Check sheet for the modelled part. Datum: model origin and axes. Units: mm. Face numbers are marked on the shaded views. A direction names the side the tool comes from. Round coordinates to 2 decimals unless told otherwise and drop trailing zeros. Order: outer loops, then holes, each group sorted by start corner. A loop starts at its lowest first (then second) coordinate and runs counter-clockwise, first axis right, second up. Notation, with made-up numbers: M -10,16.25 L 7,16.25 A24 ccw 7,31.25 Z; hole C 20,82.5 d3. An arc over 180 degrees is marked long. One line per item, written item: value. Start each with the question number.
(1) Release check for a two-part mould opening along Y. For the marked faces 5, 6 and 7 record: released by +Y, released by -Y, zero draft, split by the parting line, or undercut.
(2) Cross-section at B-B, the plane y = 6.5. Count the separate pieces of the cut face and the enclosed holes in it, and give its area (3 significant figures).
(3) Cross-section at A-A, the plane x = -17. Enter the section's corners in (y, z).
(4) Access from +Z, -Z, +X, -X, +Y, -Y to the whole of each face (thin tool, end or side, straight path). Record for the marked faces 1, 2, 3 and 4.
(5) Thickness scan on L1, parallel to Z at x = 2.65, y = 0; L2, parallel to Y at x = -3.4, z = 29.5; L3, parallel to Y at x = 38, z = 1. Record the ranges inside material, lowest first.
(6) Depth check by flat-ended pin: pin 1 Ø8 at (y, z) = (2, 11.5) entering from +X; pin 2 Ø8 at (y, z) = (2, 31.5) entering from -X; pin 3 Ø5 at (y, z) = (-3, 10) entering from -X. Enter the tip coordinate at first touch or a pass-through.
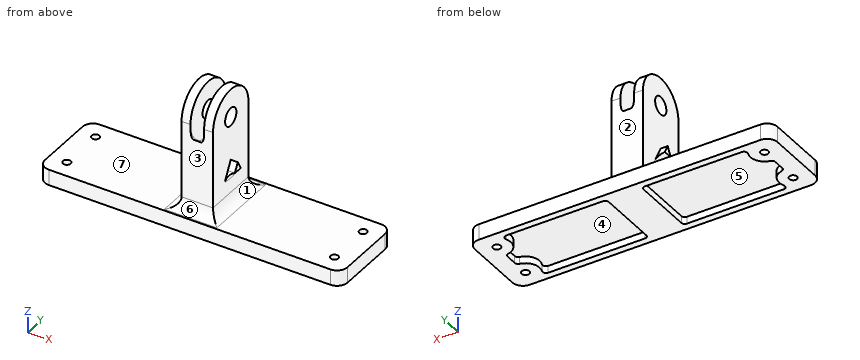
from build123d import *

# Parameters (mm, degrees)
SKETCH1_W           = 86.5
SKETCH1_H           = 23
SKETCH1_R           = 1.1
BOSS_EXTRUDE1_DEPTH = 4.5
CUT_EXTRUDE1_DEPTH  = 2
SKETCH3_R           = 2.55
BOSS_EXTRUDE2_DEPTH = 4.5
SKETCH6_R           = 9
CUT_EXTRUDE3_DEPTH  = 1.95
FILLET1_R           = 3
FILLET2_R           = 1
FILLET3_R           = 1
BOSS_EXTRUDE3_DEPTH = 2
FILLET4_R           = 3


with BuildPart() as part:
    # Sketch1 → Boss-Extrude1 (new body)
    with BuildSketch(Plane.XY):
        Rectangle(SKETCH1_W, SKETCH1_H)
        with Locations((38.25, 6.5)):
            Circle(SKETCH1_R, mode=Mode.SUBTRACT)
        with Locations((38.25, -6.5)):
            Circle(SKETCH1_R, mode=Mode.SUBTRACT)
        with Locations((-38.25, -6.5)):
            Circle(SKETCH1_R, mode=Mode.SUBTRACT)
        with Locations((-38.25, 6.5)):
            Circle(SKETCH1_R, mode=Mode.SUBTRACT)
    extrude(amount=BOSS_EXTRUDE1_DEPTH)

    # Sketch2 → Cut-Extrude1 (cut)
    with BuildSketch(Plane(origin=(0, 0, 0), x_dir=(-1, 0, 0), z_dir=(0, 0, -1))):
        with BuildLine():
            Line((-5, 9.5), (-35.604248689, 9.5))
            ThreePointArc((-35.604248689, 9.5), (-34.508342613, 5.085786438), (-38.25, 2.5))
            Line((-38.25, 2.5), (-38.25, -2.5))
            ThreePointArc((-38.25, -2.5), (-34.508342613, -5.085786438), (-35.604248689, -9.5))
            Line((-35.604248689, -9.5), (-5, -9.5))
            Line((-5, -9.5), (-5, 9.5))
        make_face()
        with BuildLine():
            Line((35.604248689, 9.5), (5, 9.5))
            Line((5, 9.5), (5, -9.5))
            Line((5, -9.5), (35.604248689, -9.5))
            ThreePointArc((35.604248689, -9.5), (34.508342613, -5.085786438), (38.25, -2.5))
            Line((38.25, -2.5), (38.25, 2.5))
            ThreePointArc((38.25, 2.5), (34.508342613, 5.085786438), (35.604248689, 9.5))
        make_face()
    extrude(amount=-CUT_EXTRUDE1_DEPTH, mode=Mode.SUBTRACT)

    # Sketch3 → Boss-Extrude2 (add, symmetric)
    with BuildSketch(Plane(origin=(0, 0, 0), x_dir=(0, 0, -1), z_dir=(1, 0, 0))):
        with BuildLine():
            Line((-29.5, 8), (-4.5, 8))
            Line((-4.5, 8), (-4.5, -8))
            Line((-4.5, -8), (-29.5, -8))
            ThreePointArc((-29.5, -8), (-37.5, 0), (-29.5, 8))
        make_face()
        with Locations((-29.5, 0)):
            Circle(SKETCH3_R, mode=Mode.SUBTRACT)
    extrude(amount=BOSS_EXTRUDE2_DEPTH, both=True)

    # Sketch6 → Cut-Extrude3 (cut, symmetric)
    with BuildSketch(Plane(origin=(0, 0, 0), x_dir=(0, 0, -1), z_dir=(1, 0, 0))):
        with Locations((-29.5, 0)):
            Circle(SKETCH6_R)
    extrude(amount=CUT_EXTRUDE3_DEPTH, both=True, mode=Mode.SUBTRACT)

    # Fillet1
    fillet1_edges = [part.edges().sort_by_distance(p)[0] for p in [
        (4.5, 0, 4.5),
        (-4.5, 0, 4.5),
        (0, -8, 4.5),
        (0, 8, 4.5),
        (43.25, -11.5, 2.25),
        (-43.25, -11.5, 2.25),
        (-43.25, 11.5, 2.25),
        (43.25, 11.5, 2.25),
    ]]
    fillet(fillet1_edges, radius=FILLET1_R)

    # Fillet2
    fillet2_edges = [part.edges().sort_by_distance(p)[0] for p in [
        (1.95, 0, 20.5),
        (-1.95, 0, 20.5),
    ]]
    fillet(fillet2_edges, radius=FILLET2_R)

    # Fillet3
    fillet3_edges = [part.edges().sort_by_distance(p)[0] for p in [
        (35.604248689, -9.5, 1),
        (38.25, -2.5, 1),
        (38.25, 2.5, 1),
        (35.604248689, 9.5, 1),
        (5, 9.5, 1),
        (5, -9.5, 1),
        (-35.604248689, -9.5, 1),
        (-5, -9.5, 1),
        (-5, 9.5, 1),
        (-35.604248689, 9.5, 1),
        (-38.25, 2.5, 1),
        (-38.25, -2.5, 1),
    ]]
    fillet(fillet3_edges, radius=FILLET3_R)

    # Sketch7 → Boss-Extrude3 (add)
    with BuildSketch(Plane(origin=(4.5, 0, 0), x_dir=(0, 0, -1), z_dir=(1, 0, 0))):
        Polygon((-14.557079529, 1.307336141), (-17, 0), (-14.557079529, 0), align=None)
        Polygon((-14.557079529, 0), (-17, 0), (-14.557079529, -1.307336141), align=None)
        with BuildLine():
            Line((-14.557079529, 0), (-14.557079529, -1.307336141))
            ThreePointArc((-14.557079529, -1.307336141), (-14.514276676, -0.65429081), (-14.5, 0))
            Line((-14.5, 0), (-14.557079529, 0))
        make_face()
        with BuildLine():
            ThreePointArc((-14.5, 0), (-14.514276676, 0.65429081), (-14.557079529, 1.307336141))
            Line((-14.557079529, 1.307336141), (-14.557079529, 0))
            Line((-14.557079529, 0), (-14.5, 0))
        make_face()
    boss_extrude3 = extrude(amount=BOSS_EXTRUDE3_DEPTH)

    # Mirror1: Boss-Extrude3 across plane
    add(boss_extrude3.mirror(Plane(origin=(0, 0, 0), x_dir=(0, 0, 1), z_dir=(1, 0, 0))))

    # Fillet4
    # the kernel refuses this fillet: 3 mm, written as the material it adds along each edge
    with BuildSketch(Plane(origin=(4.5, 0, 29.5), x_dir=(0, -0.5300616948891074, -0.8479590789721441), z_dir=(0, -0.8479590789721441, 0.5300616948891074))) as fillet4_piece_1_section:
        with BuildLine():
            CenterArc((17.828427125, 3), FILLET4_R, 199.471220634, 70.528779366)
            Line((15, 2), (14.943431458, 1.98))
            ThreePointArc((14.943431458, 1.98), (14.94, 1), (14.94, 0))
            Line((14.94, 0), (15, -0.06))
            Line((15, -0.06), (17.828427125, -0.06))
            Line((17.828427125, -0.06), (17.828427125, 0))
        make_face()
    fillet4_piece_1 = revolve(axis=Axis((4.5, 0, 29.5), (1, 0, 0)), revolution_arc=64.019246795, mode=Mode.PRIVATE)
    fillet4_piece_1 = split(fillet4_piece_1, bisect_by=Plane(origin=(4.960273163, -1.358360802, 14.461733593), z_dir=(0, 0.8816858925187555, -0.47183682235854135)), keep=Keep.TOP, mode=Mode.PRIVATE)
    fillet4_piece_1 = split(fillet4_piece_1, bisect_by=Plane(origin=(4.960273163, 1.358360693, 14.461733796), z_dir=(0, -0.8816858925186548, -0.4718368223587294)), keep=Keep.TOP, mode=Mode.PRIVATE)
    add(fillet4_piece_1)
    with BuildSketch(Plane(origin=(-4.5, 0, 29.5), x_dir=(0, -0.5300616948891074, -0.8479590789721441), z_dir=(0, -0.8479590789721441, 0.5300616948891074))) as fillet4_piece_2_section:
        with BuildLine():
            CenterArc((17.828427125, -3), FILLET4_R, 90, 70.528779366)
            Line((15, -2), (14.943431458, -1.98))
            ThreePointArc((14.943431458, -1.98), (14.94, -1), (14.94, 0))
            Line((14.94, 0), (15, 0.06))
            Line((15, 0.06), (17.828427125, 0.06))
            Line((17.828427125, 0.06), (17.828427125, 0))
        make_face()
    fillet4_piece_2 = revolve(axis=Axis((-4.5, 0, 29.5), (1, 0, 0)), revolution_arc=64.019246795, mode=Mode.PRIVATE)
    fillet4_piece_2 = split(fillet4_piece_2, bisect_by=Plane(origin=(-4.960273163, -1.358360802, 14.461733593), z_dir=(0, 0.8816858925187555, -0.47183682235854135)), keep=Keep.TOP, mode=Mode.PRIVATE)
    fillet4_piece_2 = split(fillet4_piece_2, bisect_by=Plane(origin=(-4.960273163, 1.358360693, 14.461733796), z_dir=(0, -0.8816858925186548, -0.4718368223587294)), keep=Keep.TOP, mode=Mode.PRIVATE)
    add(fillet4_piece_2)


solid = part.part
Values found:
1. face 5: undercut
1. face 6: released by -Y
1. face 7: zero draft
2. separate pieces: 3
2. enclosed holes: 0
2. area: 481 mm^2
3. outline: M -11.5,0 L -9.5,0 L -9.5,2 L 9.5,2 L 9.5,0 L 11.5,0 L 11.5,4.5 L -11.5,4.5 Z
4. face 1: +X, +Y, -Y
4. face 2: +Z, +X, -X, +Y
4. face 3: +Z, +X, -X, -Y
4. face 4: -Z
5. L1: 0 to 26.95, 32.05 to 37.5
5. L2: -8 to -2.55, 2.55 to 8
5. L3: -11.5 to -7.57, -5.43 to -2.26, 2.26 to 5.43, 7.57 to 11.5
6. pin 1: x = 6.5
6. pin 2: x = -4.5
6. pin 3: x = -4.56
